Source: three-view drawing plus pictorial views. Frame: mm from the lowest corner of the part. A direction names the side the tool comes from. Coordinates: 2 decimals unless noted, no trailing zeros. Write each loop counter-clockwise with the first axis right and the second up, starting at its lowest first coordinate (ties: lowest second). Pieces come first, ordered by that corner, then holes. Notation, with made-up numbers: M -28,57.5 L 16,57.5 A10 cw 16,70.5 Z; hole C 2.25,5.5 d4. An arc over 180 degrees is marked long. Answer as a JSON object with one key per item and string values. Group by question number.
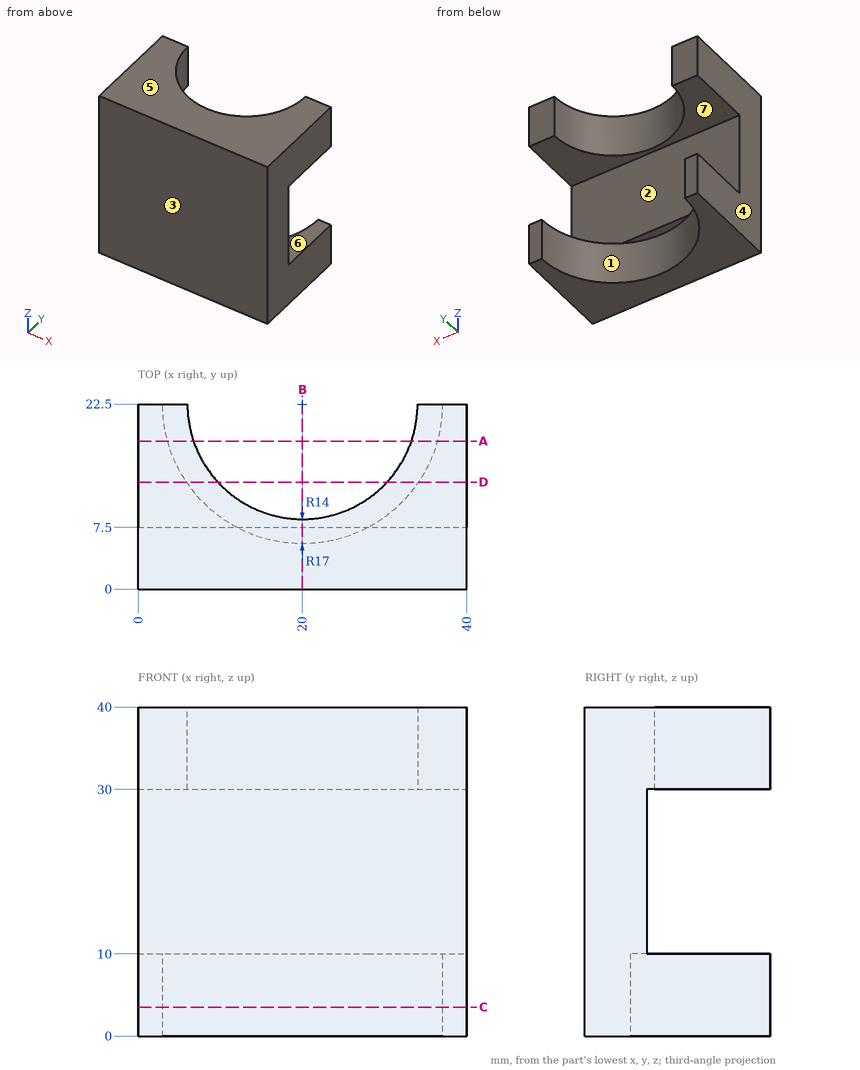
Q1. Draft query along Z for the marked faces 4, 5, 6 and 7. Return one class per face: released by +Z, released by -Z, zero draft, split by the parting line, or undercut.
Q2. Access query for the marked faces 1, 2 and 3. Directions: +Z, -Z, +X, -X, +Y, -Y. A direction counts if a zero-diameter tool reaches every point of the face in a straight line with its end or side. Return the directions, or none.
Q3. Pin query (flat end, axial travel): pin 1 Ø1.5 at (y, z) = (11.5, 29) entering from +X; pin 2 Ø6 at (x, z) = (12.5, 34.5) entering from +Y; pin 3 Ø22 at (x, z) = (18.5, 24) entering from +Y; pin 4 Ø8 at (x, y) = (29.5, 16) entering from -Z. Return the tip coordinate at first contact, or that it passes through.
Q4. Section C-C, the plane z = 3.5. Return the cut outline in (x, y).
Q5. Section B-B, the plane x = 20. Return the cut outline in (y, z).
Q6. Section A-A, the plane y = 18. Return the cut outline in (x, z), and give its area (3 significant figures).
Q7. Line query: line 1 (Z direction, x = 34, y = 8.75); line 2 (X direction, y = 16.5, z = 33); line 3 (X direction, y = 13.75, z = 8.5). Output: solid intervals per line, ascending. Write a range as from..to.
Q8. Section D-D, the plane y = 13. Return the cut outline in (x, z), and give its area (3 significant figures).
Filled in:
{
 "1": {"face 4": "zero draft", "face 5": "released by +Z", "face 6": "undercut", "face 7": "undercut"},
 "2": {"face 1": "-Z, +Y", "face 2": "+X, -X, +Y", "face 3": "+Z, -Z, +X, -X, -Y"},
 "3": {"pin 1": "through", "pin 2": "y = 13.24", "pin 3": "y = 13.49", "pin 4": "z = 30"},
 "4": {"outline": "M 0,0 L 40,0 L 40,22.5 L 37,22.5 A17 cw 3,22.5 L 0,22.5 Z"},
 "5": {"outline": "M 0,0 L 5.5,0 L 5.5,10 L 7.5,10 L 7.5,30 L 8.5,30 L 8.5,40 L 0,40 Z"},
 "6": {"outline": "M 0,0 L 3.61,0 L 3.61,10 L 0,10 Z; M 0,30 L 6.74,30 L 6.74,40 L 0,40 Z; M 33.26,30 L 40,30 L 40,40 L 33.26,40 Z; M 36.39,0 L 40,0 L 40,10 L 36.39,10 Z", "area": "207 mm^2"},
 "7": {"line 1": "0..10, 30..40", "line 2": "0..7.35, 32.65..40", "line 3": "0..5.42, 34.58..40"},
 "8": {"outline": "M 0,0 L 5.9,0 L 5.9,10 L 0,10 Z; M 0,30 L 9.72,30 L 9.72,40 L 0,40 Z; M 30.28,30 L 40,30 L 40,40 L 30.28,40 Z; M 34.1,0 L 40,0 L 40,10 L 34.1,10 Z", "area": "312 mm^2"}
}
